Source: CAD feature listing. Evaluate the final solid. Frame: model axes, mm. A direction names the side the tool comes from. Give positions to 0.01 mm unless a question says otherwise; leave off trailing zeros. Loops run counter-clockwise (first coordinate to the right, second up) from the corner with the lowest first, then second, coordinate; pieces in that order, holes last. Notation, with made-up numbers: (-39, -18) -> (19, -18) arc R23 cw to (19, 8) -> close; hole circle Ø9 at (26, -13.5). An arc over 180 degrees is marked (long way). Return JSON: item names as keys, results as strings. Group by question number.
(1) Ray query, line 1 (Z direction, x = -25.5, y = 6); line 2 (X direction, y = 36, z = -8.25); line 3 (Y direction, x = -23, z = 4.5). Return the intervals inside material, ascending. Write a range as from..to.
(2) Draft query along X for faces 4 (the face through (0, 16, -10)), 5 (the face through (29, 16, -9)), 6 (the face through (22.5, 32, -9)). Return one class per face: released by +X, released by -X, zero draft, split by the parting line, or undercut.
(3) Access query for faces 1 (the face through (0, 17, -8)), 2 (the face through (-26, 42, -9)), 3 (the face through (-22.5, 32, -9)). Directions: +Z, -Z, +X, -X, +Y, -Y. A direction counts if a zero-diameter tool reaches every point of the face in a straight line with its end or side. Return the directions, or none.
(4) Cut plane D-D on y = 7.5. Return loops of the section in (x, z).
(5) Cut plane A-A on y = 32.5. Return loops of the section in (x, z), then the cut area to 3 significant figures.
(6) Cut plane C-C on x = -15.5. Return loops of the section in (y, z), then the cut area to 3 significant figures.
(7) Cut plane B-B on z = -9. Return loops of the section in (x, y).
(8) Pin query (flat end, axial travel): pin 1 (1.5 mm diameter, centred on x = 20.5, y = 9, fed in from +Z); pin 2 (1.6 mm diameter, centred on x = 5, z = -9, fed in from +Y); pin 3 (6 mm diameter, centred on x = 13.5, z = 2, fed in from +Y). Return the tip coordinate at first contact, or that it passes through.
```python
from build123d import *

# Parameters (mm, degrees)
SKETCH1_W           = 58
SKETCH1_H           = 20
BOSS_EXTRUDE1_DEPTH = 2
SKETCH2_W           = 58
SKETCH2_H           = 2
BOSS_EXTRUDE2_DEPTH = 40
SKETCH3_W           = 45
SKETCH3_H           = 20
CUT_EXTRUDE1_DEPTH  = 60


with BuildPart() as part:
    # Sketch1 → Boss-Extrude1 (new body)
    with BuildSketch(Plane(origin=(0, 0, 0), x_dir=(1, 0, 0), z_dir=(0, 1, 0))):
        Rectangle(SKETCH1_W, SKETCH1_H)
    extrude(amount=BOSS_EXTRUDE1_DEPTH)

    # Sketch2 → Boss-Extrude2 (add)
    with BuildSketch(Plane(origin=(0, 2, 0), x_dir=(1, 0, 0), z_dir=(0, 1, 0))):
        with Locations((0, 9)):
            Rectangle(SKETCH2_W, SKETCH2_H)
    extrude(amount=BOSS_EXTRUDE2_DEPTH)

    # Sketch3 → Cut-Extrude1 (cut)
    with BuildSketch(Plane.XY.offset(-8)):
        with Locations((0, 32)):
            Rectangle(SKETCH3_W, SKETCH3_H)
    extrude(amount=-CUT_EXTRUDE1_DEPTH, mode=Mode.SUBTRACT)


solid = part.part
```
Answers:
{
 "1": {"line 1": "-10..-8", "line 2": "-29..-22.5, 22.5..29", "line 3": "0..2"},
 "2": {"face 4": "zero draft", "face 5": "released by +X", "face 6": "undercut"},
 "3": {"face 1": "+Z, +X, -X, +Y", "face 2": "+Z, -Z, +X, -X, +Y", "face 3": "+Z, -Z, +Y"},
 "4": {"outline": "(-29, -10) -> (29, -10) -> (29, -8) -> (-29, -8) -> close"},
 "5": {"outline": "(-29, -10) -> (-22.5, -10) -> (-22.5, -8) -> (-29, -8) -> close; (22.5, -10) -> (29, -10) -> (29, -8) -> (22.5, -8) -> close", "area": "26.0 mm²"},
 "6": {"outline": "(0, -10) -> (22, -10) -> (22, -8) -> (2, -8) -> (2, 10) -> (0, 10) -> close", "area": "80.0 mm²"},
 "7": {"outline": "(-29, 0) -> (29, 0) -> (29, 42) -> (22.5, 42) -> (22.5, 22) -> (-22.5, 22) -> (-22.5, 42) -> (-29, 42) -> close"},
 "8": {"pin 1": "z = -8", "pin 2": "y = 22", "pin 3": "y = 2"}
}
